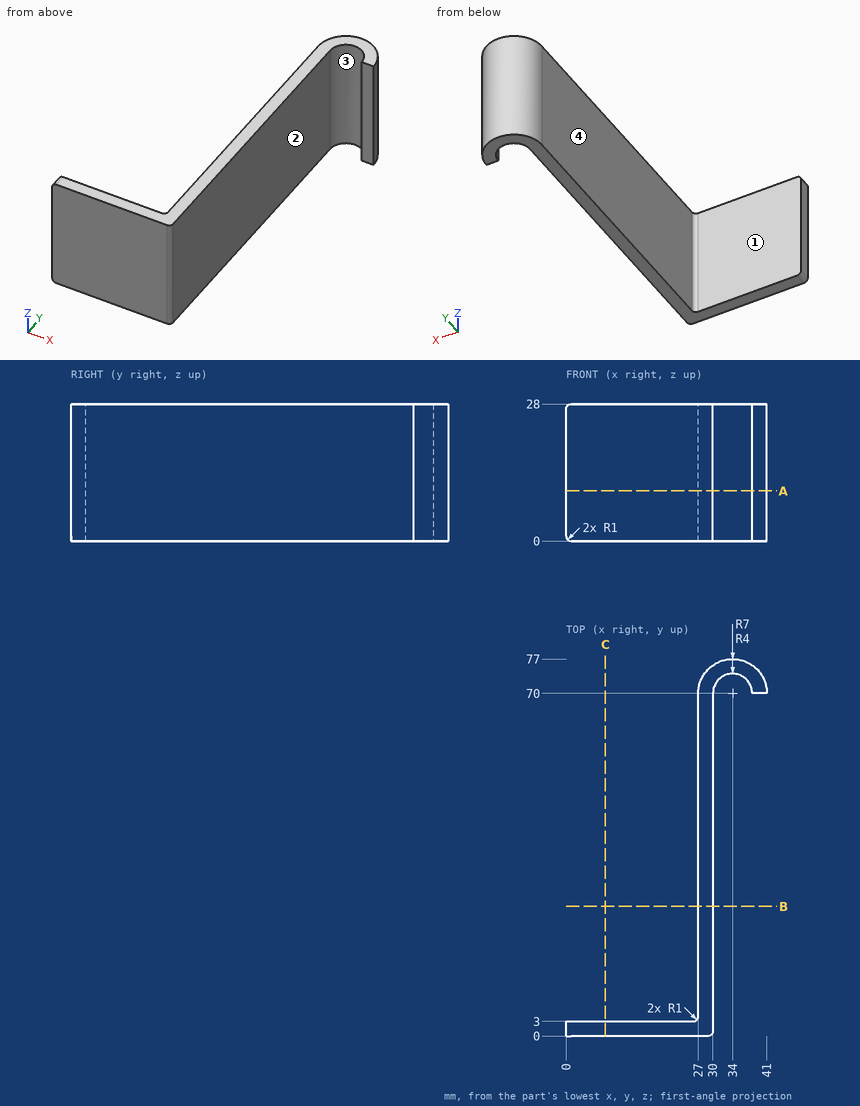
Can you work these out from the drawing? Everything is in mm from the part's minimum corner. Give positions to 0.01 mm unless a question says otherwise; leave off trailing zeros. Loops run counter-clockwise (first coordinate to the right, second up) from the corner with the lowest first, then second, coordinate; pieces in that order, holes last. Notation, with made-up numbers: M 11,58.5 L 45,58.5 A19 ccw 45,67.5 Z; hole C 71.5,54 d6. An arc over 180 degrees is marked long. Put each result on its own line as item: value. Start each with the question number.
(1) I want a section at A-A on z = 10.25. Please give me the cut outline in (x, y), then the cut area to 3 significant figures.
(2) Will these pins go through, and if not, where does the flat tip stop? pin 1 Ø8.5 at (y, z) = (31, 10.5) entering from -X; pin 2 Ø1.5 at (x, z) = (13, 11.5) entering from +Y; pin 3 Ø6 at (x, z) = (36, 18) entering from -Y.
(3) If we mould it in two halves opening along X, with no side actions, what happens to the marked faces 1, 2, 3 and 4? For each: +X half, -X half, draft (parallel to the pull), parting line (faces both ways), or undercut.
(4) I need wall thicknesses on line 1 along Y through (x, z) = (3.5, 14.5); line 2 along X through (y, z) = (5.5, 8); line 3 along Y through (x, z) = (28.5, 5.5). Which ranges of each line are inside material? Lowest first, please. Write a range as [from, to].
(5) I want a section at B-B on y = 26.5. Please give me the cut outline in (x, z).
(6) I want a section at C-C on x = 8. Please give me the cut outline in (y, z).
Answer block:
1. outline: M 0,0 L 29,0 A1 ccw 30,1 L 30,70 A4 cw 38,70 L 41,70 A7 ccw 27,70 L 27,4 A1 cw 26,3 L 0,3 Z
1. area: 343 mm^2
2. pin 1: x = 27
2. pin 2: y = 3
2. pin 3: y = 70
3. face 1: draft
3. face 2: +X half
3. face 3: undercut
3. face 4: -X half
4. line 1: [0, 3]
4. line 2: [27, 30]
4. line 3: [0, 74.33]
5. outline: M 27,0 L 30,0 L 30,28 L 27,28 Z
6. outline: M 0,0 L 3,0 L 3,28 L 0,28 Z
